Autodesk Inventor part; units mm, degrees
ref_plane "XZ Plane" through (0, 0, 0) normal (0, 1, 0) x (-1, 0, 0)
sketch "Sketch1" plane through (0, 0, 0) normal (0, 1, 0) x (-1, 0, 0)
  line L0 (-10.577, 9.85) -> (-48.827, 9.85) construction
  arc A0 (-9.577, 8.85) -> (-10.577, 9.85) centre (-10.577, 8.85) ccw construction
  line L1 (-9.577, -8.85) -> (-9.577, 8.85) construction
  arc A1 (-10.577, -9.85) -> (-9.577, -8.85) centre (-10.577, -8.85) ccw construction
  line L2 (-48.827, -9.85) -> (-10.577, -9.85) construction
  arc A2 (-49.827, -8.85) -> (-48.827, -9.85) centre (-48.827, -8.85) ccw construction
  line L3 (-49.827, 8.85) -> (-49.827, -8.85) construction
  arc A3 (-48.827, 9.85) -> (-49.827, 8.85) centre (-48.827, 8.85) ccw construction
  circle A4 centre (-19.427, 0) radius 6.44 construction
  circle A5 centre (-19.427, 0) radius 5.44 construction
  line L4 (-9.577, 9.475) -> (-3.217, 9.475) construction
  arc A6 (-2.217, 8.475) -> (-3.217, 9.475) centre (-3.217, 8.475) ccw construction
  line L5 (-2.217, -8.475) -> (-2.217, 8.475) construction
  arc A7 (-3.217, -9.475) -> (-2.217, -8.475) centre (-3.217, -8.475) ccw construction
  line L6 (-9.577, -9.475) -> (-3.217, -9.475) construction
  circle A8 centre (-5.6393, -4.36) radius 2.3 construction
  circle A9 centre (-5.6393, 4.36) radius 2.18 construction
  line L7 (-49.6076, 9.475) -> (-56.187, 9.475) construction
  arc A10 (-56.187, 9.475) -> (-57.187, 8.475) centre (-56.187, 8.475) ccw construction
  line L8 (-57.187, -8.475) -> (-57.187, 8.475) construction
  circle A11 centre (-53.7647, 4.36) radius 2.18 construction
  circle A12 centre (-53.7647, -4.36) radius 2.3 construction
  line L9 (-56.187, -9.475) -> (-49.6076, -9.475) construction
  arc A13 (-57.187, -8.475) -> (-56.187, -9.475) centre (-56.187, -8.475) ccw construction
  line L10 (48.9003, 9.85) -> (10.6503, 9.85) construction
  arc A14 (49.9003, 8.85) -> (48.9003, 9.85) centre (48.9003, 8.85) ccw construction
  line L11 (49.9003, -8.85) -> (49.9003, 8.85) construction
  arc A15 (48.9003, -9.85) -> (49.9003, -8.85) centre (48.9003, -8.85) ccw construction
  line L12 (10.6503, -9.85) -> (48.9003, -9.85) construction
  arc A16 (9.6503, -8.85) -> (10.6503, -9.85) centre (10.6503, -8.85) ccw construction
  line L13 (9.6503, 8.85) -> (9.6503, -8.85) construction
  arc A17 (10.6503, 9.85) -> (9.6503, 8.85) centre (10.6503, 8.85) ccw construction
  circle A18 centre (40.0503, 0) radius 6.44 construction
  circle A19 centre (40.0503, 0) radius 5.44 construction
  line L14 (49.9003, 9.475) -> (56.2603, 9.475) construction
  arc A20 (57.2603, 8.475) -> (56.2603, 9.475) centre (56.2603, 8.475) ccw construction
  line L15 (57.2603, -8.475) -> (57.2603, 8.475) construction
  arc A21 (56.2603, -9.475) -> (57.2603, -8.475) centre (56.2603, -8.475) ccw construction
  line L16 (49.9003, -9.475) -> (56.2603, -9.475) construction
  circle A22 centre (53.838, -4.36) radius 2.3 construction
  circle A23 centre (53.838, 4.36) radius 2.18 construction
  line L17 (9.8697, 9.475) -> (3.2903, 9.475) construction
  arc A24 (3.2903, 9.475) -> (2.2903, 8.475) centre (3.2903, 8.475) ccw construction
  line L18 (2.2903, -8.475) -> (2.2903, 8.475) construction
  circle A25 centre (5.7126, 4.36) radius 2.18 construction
  circle A26 centre (5.7126, -4.36) radius 2.3 construction
  line L19 (3.2903, -9.475) -> (9.8697, -9.475) construction
  arc A27 (2.2903, -8.475) -> (3.2903, -9.475) centre (3.2903, -8.475) ccw construction
  line L20 (-62.7873, 21.97) -> (62.7873, 21.97)
  line L21 (62.7873, 21.97) -> (62.7873, -21.97)
  line L22 (62.7873, -21.97) -> (-62.7873, -21.97)
  line L23 (-62.7873, -21.97) -> (-62.7873, 21.97)
  line L24 (-62.7873, 21.97) -> (62.7873, -21.97) construction
  line L25 (62.7873, 21.97) -> (-62.7873, -21.97) construction
  point P0 (0, 0)
extrude "Socle" add sketch "Sketch1" along normal blind 30
sketch "Sketch2" plane through (0, 30, 0) normal (0, 1, 0) x (1, 0, 0)
  line L0 (-10.577, 9.85) -> (-48.827, 9.85)
  arc A0 (-9.577, 8.85) -> (-10.577, 9.85) centre (-10.577, 8.85) ccw
  line L1 (-9.577, -8.85) -> (-9.577, 8.85)
  arc A1 (-10.577, -9.85) -> (-9.577, -8.85) centre (-10.577, -8.85) ccw
  line L2 (-48.827, -9.85) -> (-10.577, -9.85)
  arc A2 (-49.827, -8.85) -> (-48.827, -9.85) centre (-48.827, -8.85) ccw
  line L3 (-49.827, 8.85) -> (-49.827, -8.85)
  arc A3 (-48.827, 9.85) -> (-49.827, 8.85) centre (-48.827, 8.85) ccw
  circle A4 centre (-19.427, 0) radius 6.44 construction
  circle A5 centre (-19.427, 0) radius 5.44 construction
  line L4 (-9.577, 9.475) -> (-3.217, 9.475) construction
  arc A6 (-2.217, 8.475) -> (-3.217, 9.475) centre (-3.217, 8.475) ccw construction
  line L5 (-2.217, -8.475) -> (-2.217, 8.475) construction
  arc A7 (-3.217, -9.475) -> (-2.217, -8.475) centre (-3.217, -8.475) ccw construction
  line L6 (-9.577, -9.475) -> (-3.217, -9.475) construction
  circle A8 centre (-5.6393, -4.36) radius 2.3
  circle A9 centre (-5.6393, 4.36) radius 2.18
  line L7 (-49.6076, 9.475) -> (-56.187, 9.475) construction
  arc A10 (-56.187, 9.475) -> (-57.187, 8.475) centre (-56.187, 8.475) ccw construction
  line L8 (-57.187, -8.475) -> (-57.187, 8.475) construction
  circle A11 centre (-53.7647, 4.36) radius 2.18
  circle A12 centre (-53.7647, -4.36) radius 2.3
  line L9 (-56.187, -9.475) -> (-49.6076, -9.475) construction
  arc A13 (-57.187, -8.475) -> (-56.187, -9.475) centre (-56.187, -8.475) ccw construction
  circle A14 centre (40.0503, 0) radius 5.44 construction
  circle A15 centre (40.0503, 0) radius 6.44 construction
  line L10 (48.9003, 9.85) -> (10.6503, 9.85)
  line L11 (10.6503, -9.85) -> (48.9003, -9.85)
  arc A16 (48.9003, -9.85) -> (49.9003, -8.85) centre (48.9003, -8.85) ccw
  arc A17 (49.9003, 8.85) -> (48.9003, 9.85) centre (48.9003, 8.85) ccw
  line L12 (49.9003, -8.85) -> (49.9003, 8.85)
  circle A18 centre (53.838, 4.36) radius 2.18
  line L13 (49.9003, 9.475) -> (56.2603, 9.475) construction
  arc A19 (57.2603, 8.475) -> (56.2603, 9.475) centre (56.2603, 8.475) ccw construction
  line L14 (57.2603, -8.475) -> (57.2603, 8.475) construction
  circle A20 centre (53.838, -4.36) radius 2.3
  line L15 (49.9003, -9.475) -> (56.2603, -9.475) construction
  arc A21 (56.2603, -9.475) -> (57.2603, -8.475) centre (56.2603, -8.475) ccw construction
  arc A22 (9.6503, -8.85) -> (10.6503, -9.85) centre (10.6503, -8.85) ccw
  line L16 (9.6503, 8.85) -> (9.6503, -8.85)
  arc A23 (10.6503, 9.85) -> (9.6503, 8.85) centre (10.6503, 8.85) ccw
  line L17 (9.8697, 9.475) -> (3.2903, 9.475) construction
  circle A24 centre (5.7126, 4.36) radius 2.18
  arc A25 (3.2903, 9.475) -> (2.2903, 8.475) centre (3.2903, 8.475) ccw construction
  line L18 (2.2903, -8.475) -> (2.2903, 8.475) construction
  circle A26 centre (5.7126, -4.36) radius 2.3
  line L19 (3.2903, -9.475) -> (9.8697, -9.475) construction
  arc A27 (2.2903, -8.475) -> (3.2903, -9.475) centre (3.2903, -8.475) ccw construction
  line L20 (-62.7873, 21.97) -> (62.7873, 21.97) construction
  line L21 (62.7873, 21.97) -> (62.7873, -21.97) construction
  line L22 (62.7873, -21.97) -> (-62.7873, -21.97) construction
  line L23 (-62.7873, -21.97) -> (-62.7873, 21.97) construction
  line L24 (-62.7873, 21.97) -> (62.7873, -21.97) construction
  line L25 (62.7873, 21.97) -> (-62.7873, -21.97) construction
  point P0 (0, 0)
  point P1 (0, 0)
  point P2 (0, 0)
extrude "empreinte" cut sketch "Sketch2" against normal blind 28
fillet "Fillet1" radius 3.175 1 edges at (-62.7873, 15, 21.97)
fillet "Fillet2" radius 3.175 1 edges at (62.7873, 15, 21.97)
fillet "Fillet3" radius 3.175 1 edges at (62.7873, 15, -21.97)
fillet "Fillet4" radius 3.175 1 edges at (-62.7873, 15, -21.97)
chamfer "Chamfer1" distance 3.175 angle 45 8 edges at (0, 30, 21.97) (61.8574, 30, 21.0401) (62.7873, 30, 0) (61.8574, 30, -21.0401) (0, 30, -21.97) (-61.8574, 30, -21.0401) (-62.7873, 30, 0) (-61.8574, 30, 21.0401)
sketch "Sketch3" plane through (-62.7873, 0, -18.795) normal (-1, 0, 0) x (0, 0, 1)
  point P0 (18.795, 0)
sketch "Sketch4" plane through (-62.7873, 0, -18.795) normal (-1, 0, 0) x (0, 0, 1)
  line L0 (-3.175, 0) -> (-3.175, 26.825)
  line L1 (0, 0) -> (-3.175, 0)
  line L2 (0, 0) -> (37.59, 0)
  line L3 (40.765, 0) -> (37.59, 0)
  line L4 (40.765, 26.825) -> (40.765, 0)
  point P0 (18.795, 0)
sketch "Sketch5" plane through (-62.7873, 0, -18.795) normal (-1, 0, 0) x (0, 0, 1)
  line L0 (12.255, 30) -> (12.255, 2) construction
  line L1 (28.758, 1.5182) -> (8.832, 1.5182)
  line L2 (8.832, 1.5182) -> (8.832, 0) construction
  line L3 (8.832, 0) -> (28.758, 0) construction
  line L4 (28.758, 0) -> (28.758, 1.5182) construction
  line L5 (28.758, 1.5182) -> (8.832, 0) construction
  line L6 (8.832, 1.5182) -> (28.758, 0) construction
  line L7 (25.455, 30) -> (25.455, 2) construction
  line L8 (8.832, 1.5182) -> (10.3503, 0)
  line L9 (8.832, 1.5182) -> (10.9792, 1.5182) construction
  line L10 (28.758, 1.5182) -> (27.2397, 0)
  line L11 (28.758, 1.5182) -> (30.9051, 1.5182) construction
  line L12 (10.3503, 0) -> (27.2397, 0) construction
  line L13 (10.3503, 0) -> (27.2397, 0)
  line L14 (37.59, 0) -> (0, 0)
  point P0 (18.795, 0)
  point P1 (18.795, 0.7591)
  dimension "d11" = 45
  dimension "d12" = 135
extrude "Extrusion3" cut sketch "Sketch5" against normal blind 125.8875
sketch "Sketch6" plane through (62.7873, 0, -18.795) normal (1, 0, 0) x (0, 0, -1)
  line L0 (-28.758, 1.5182) -> (-8.832, 1.5182)
  line L1 (-8.832, 1.5182) -> (-10.3503, 0)
  line L2 (0, 0) -> (-10.3503, 0)
  line L3 (3.175, 0) -> (0, 0)
  line L4 (3.175, 0) -> (3.175, 26.825)
  line L5 (0, 30) -> (3.175, 26.825)
  line L6 (0, 30) -> (-37.59, 30)
  line L7 (-40.765, 26.825) -> (-37.59, 30)
  line L8 (-40.765, 26.825) -> (-40.765, 0)
  line L9 (-37.59, 0) -> (-40.765, 0)
  line L10 (-27.2397, 0) -> (-37.59, 0)
  line L11 (-9.945, 30) -> (-9.945, 2)
  line L12 (-28.645, 30) -> (-28.645, 2)
  line L13 (-27.2397, 0) -> (-28.758, 1.5182)
  point P0 (-18.795, 0)
sketch "Sketch7" plane through (59.6123, 0, -21.97) normal (0, 0, -1) x (-1, 0, 0)
  point P0 (59.6123, 0)
sketch "Sketch8" plane through (0, 30, 0) normal (0, 1, 0) x (1, 0, 0)
  line L0 (9.6503, -8.85) -> (9.6503, 8.85)
  line L1 (10.6503, 9.85) -> (48.9003, 9.85)
  line L2 (48.9003, -9.85) -> (10.6503, -9.85)
  line L3 (59.6123, -18.795) -> (-59.6123, -18.795)
  line L4 (-59.6123, -21.97) -> (59.6123, -21.97)
  line L5 (62.7873, 18.795) -> (62.7873, -18.795)
  line L6 (62.7873, -21.97) -> (62.7873, -18.795)
  line L7 (59.6123, 21.97) -> (-59.6123, 21.97)
  line L8 (-62.7873, 18.795) -> (-62.7873, -18.795)
  arc A0 (-59.6123, 21.97) -> (-62.7873, 18.795) centre (-59.6123, 18.795) ccw
  arc A1 (-62.7873, -18.795) -> (-59.6123, -21.97) centre (-59.6123, -18.795) ccw
  arc A2 (62.7873, 18.795) -> (59.6123, 21.97) centre (59.6123, 18.795) ccw
  line L9 (-10.577, -9.85) -> (-48.827, -9.85)
  point P0 (0, 0)
properties part number "Socle servo"
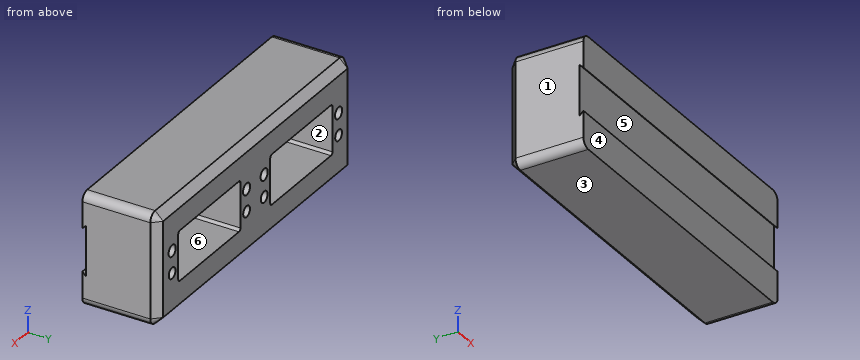
Can you work these out from the model? Positions are in its coordinate system, mm. Face numbers are marked on the shaded views. A direction names the side the tool comes from. Round coordinates to 2 decimals unless told otherwise and drop trailing zeros. Loops run counter-clockwise (first coordinate to the right, second up) from the corner with the lowest first, then second, coordinate; pieces in that order, holes last. Notation, with made-up numbers: (-8.5, -3) - (21.5, -3) arc R10 cw to (21.5, 6) - close; hole circle Ø11 at (34.5, 21.5). An arc over 180 degrees is marked (long way). Use CSV: the item, a comma, the result in double quotes. Start each with the question number.
1) For the marked faces 4, 5 and 6, which set-ups out of +Z, -Z, +X, -X, +Y, -Y let a thin tool reach every point of the face, with its end or its side?
2) We'd pull the mould along X, two halves only. Please class the marked faces 1, 2 and 3: released by +X, released by -X, zero draft, split by the parting line, or undercut.
3) If we section it at A-A on y = 12: Count the separate pieces of the cut face and the enclosed holes in it, plus the area to 3 significant figures.
4) If we section it at C-C on x = 17: Write out the boundary of the cut face in (y, z) (3 decimals), plus the area to 3 significant figures.
5) For pin 1 Ø4 at (x, z) = (-5.64, 4.36) entering from -Y; pin 2 Ø1.3 at (x, z) = (53, -4.5) entering from +Y, each with a flat end and sliding along its axis, tell me the tip position at first contact or that it passes through.
6) Please list where these lines run through material, in increasing order: probe 1 along Z at (x, y) = (54, 8); probe 2 along Z at (x, y) = (-6.5, 24.5); probe 3 along Z at (x, y) = (12.5, 23). Write a range as [from, to].
Geometry results:
1,face 4,"+Z, -Z, +X, -X, -Y"
1,face 5,"+X, -X"
1,face 6,"+Y"
2,face 1,"released by -X"
2,face 2,"undercut"
2,face 3,"zero draft"
3,separate pieces,"1"
3,enclosed holes,"10"
3,area,"3,800 mm2"
4,outline,"(0, -21.97) - (26.825, -21.97) - (30, -18.795) - (30, -9.85) - (2, -9.85) - (2, 9.85) - (30, 9.85) - (30, 18.795) - (26.825, 21.97) - (0, 21.97) - (0, 8.445) - (1.518, 9.963) - (1.518, -9.963) - (0, -8.445) - close"
4,area,"729 mm2"
5,pin 1,"stops at y = 1.52"
5,pin 2,"stops at y = 2"
6,probe 1,"z = [-21.97, -6.53], [-2.19, 2.07], [6.65, 21.97]"
6,probe 2,"z = [-21.97, -6.36], [-2.36, 2.23], [6.49, 21.97]"
6,probe 3,"z = [-21.97, -9.85], [9.85, 21.97]"
